```python
from build123d import *

# Parameters (mm, degrees)
BOSS_EXTRUDE2_REACH            = 37.012
BOSS_EXTRUDE2_END_MAJOR_RADIUS = 17.132631579
BOSS_EXTRUDE2_END_MINOR_RADIUS = 5.617368421
SKETCH4_W                      = 2
SKETCH4_H                      = 2
CIRPATTERN2_COUNT              = 3


with BuildPart() as part:
    # Sketch3 → Revolve1 (revolve)
    with BuildSketch(Plane.XY, mode=Mode.PRIVATE) as revolve1_sk:
        with BuildLine():
            Line((-24.25, 0), (-24.25, -1))
            ThreePointArc((-24.25, -1), (-22.452699724, -5.636404857), (-18, -7.85))
            Line((-18, -7.85), (0, -7.85))
            Line((0, -7.85), (0, -3.85))
            Line((0, -3.85), (-3.5, -3.85))
            Line((-3.5, -3.85), (-3.5, -6.35))
            Line((-3.5, -6.35), (-18, -6.35))
            ThreePointArc((-18, -6.35), (-21.400368447, -4.45256759), (-22.75, -0.8))
            Line((-22.75, -0.8), (-22.75, 0))
            Line((-22.75, 0), (-24.25, 0))
        make_face()
    revolve(revolve1_sk.sketch.rotate(Axis((0, -13.198525541, 0), (0, 1, 0)), 180), axis=Axis((0, -13.198525541, 0), (0, 1, 0)))

    # Boss-Extrude2: up to this torus (the profile starts inside it)
    boss_extrude2_end = Plane(origin=(0, -0.8, 0), z_dir=(0, -1, 0)) * Torus(BOSS_EXTRUDE2_END_MAJOR_RADIUS, BOSS_EXTRUDE2_END_MINOR_RADIUS, mode=Mode.PRIVATE)
    # Sketch4 → Boss-Extrude2 (add, up to the surface)
    with BuildSketch(Plane(origin=(0, -0.8, 0), x_dir=(1, 0, 0), z_dir=(0, 1, 0)), mode=Mode.PRIVATE) as boss_extrude2_sk1:
        with Locations((-21.75, 0)):
            Rectangle(SKETCH4_W, SKETCH4_H)
    boss_extrude2_tool1 = extrude(boss_extrude2_sk1.sketch, amount=-BOSS_EXTRUDE2_REACH, mode=Mode.PRIVATE) & boss_extrude2_end
    boss_extrude2 = boss_extrude2_tool1.solids().sort_by_distance((-21.75, -0.8, 0))[0]
    add(boss_extrude2)

    # CirPattern2: Boss-Extrude2 ×3 about axis
    cirpattern2_axis = Axis((0, 0, 0), (0, 1, 0))
    for i in range(1, CIRPATTERN2_COUNT):
        add(boss_extrude2.rotate(cirpattern2_axis, i * 360 / CIRPATTERN2_COUNT))


solid = part.part
```
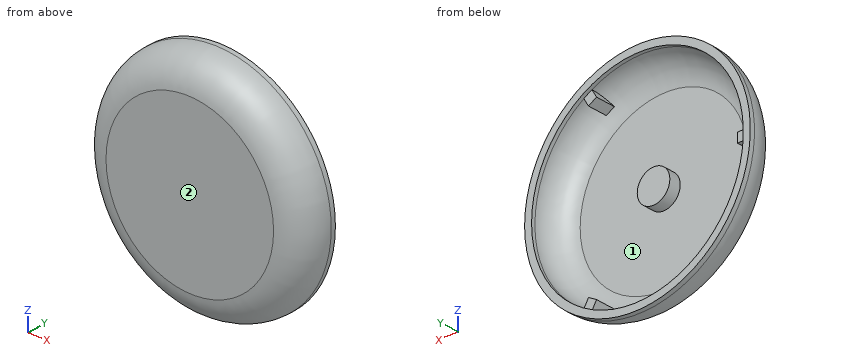
Geometry: final body of the model. Coordinates: model frame, mm. Face numbers are marked on the shaded views. A direction names the side the tool comes from. Give positions to 0.01 mm unless a question says otherwise; leave off trailing zeros. Loops run counter-clockwise (first coordinate to the right, second up) from the corner with the lowest first, then second, coordinate; pieces in that order, holes last. Notation, with made-up numbers: (29.5, -13.75) -> (57.5, -13.75) arc R11 ccw to (57.5, -4.75) -> close; hole circle Ø7 at (-16.5, 81). An arc over 180 degrees is marked (long way). Use CSV: the item, a comma, the result in double quotes.
(1) Access query for the marked faces 1 and 2. Directions: +Z, -Z, +X, -X, +Y, -Y. A direction counts if a zero-diameter tool reaches every point of the face in a straight line with its end or side. Return the directions, or none.
From the geometry:
face 1,"+Y"
face 2,"+Z, -Z, +X, -X, -Y"
(2) Cut plane B-B (y = -1.75). Output: boundary loops of the cut face in (x, z).
From the geometry:
outline,"circle Ø48.42 at (0, 0); hole (-22.65, -1) arc R22.67 ccw to (10.46, -20.11) -> (9.51, -18.47) -> (11.24, -17.47) -> (12.19, -19.11) arc R22.67 ccw to (12.19, 19.11) -> (11.24, 17.47) -> (9.51, 18.47) -> (10.46, 20.11) arc R22.67 ccw to (-22.65, 1) -> (-20.75, 1) -> (-20.75, -1) -> close"
(3) Cut plane A-A (x = 0). Output: boundary loops of the cut face in (y, z), plus the area to 3 significant figures.
From the geometry:
outline,"(-7.85, -18) arc R6.88 ccw to (-1, -24.25) -> (0, -24.25) -> (0, -22.75) -> (-0.8, -22.75) arc R5.62 cw to (-6.35, -18) -> (-6.35, -3.5) -> (-3.85, -3.5) -> (-3.85, 3.5) -> (-6.35, 3.5) -> (-6.35, 18) arc R5.62 cw to (-0.8, 22.75) -> (0, 22.75) -> (0, 24.25) -> (-1, 24.25) arc R6.88 ccw to (-7.85, 18) -> close"
area,"102 mm^2"
(4) First-contact query: P1, Ø2, axis at x = -21.5, z = 0, coming from the +Y side; P2, Ø5.5, axis at x = 1, z = 1, coming from the +Y side; P3, Ø1.6, axis at y = -2, z = 0, coming from the +X side. Flat tips, straight axial feed; report the tip coordinate or a pass-through.
From the geometry:
P1,"y = -0.8"
P2,"y = -3.85"
P3,"x = 24.25"
(5) Cut plane C-C (z = 0). Output: boundary loops of the cut face in (x, y).
From the geometry:
outline,"(-24.25, -1) arc R6.88 ccw to (-18, -7.85) -> (18, -7.85) arc R6.88 ccw to (24.25, -1) -> (24.25, 0) -> (22.75, 0) -> (22.75, -0.8) arc R5.62 cw to (18, -6.35) -> (3.5, -6.35) -> (3.5, -3.85) -> (-3.5, -3.85) -> (-3.5, -6.35) -> (-18, -6.35) arc R5.62 cw to (-20.75, -5.1) -> (-20.75, -0.8) -> (-22.75, -0.8) -> (-22.75, 0) -> (-24.25, 0) -> close"
(6) Ray query, line 1 along Z through (x, y) = (0, -0.4); line 2 along X through (y, z) = (-4, 18); line 3 along Y through (x, z) = (8, 7). Return the intervals inside material, ascending. Write a range as [from, to].
From the geometry:
line 1,"[-24.25, -22.75], [22.75, 24.25]"
line 2,"[-15.2, -12.21], [10.32, 11.55], [12.21, 15.2]"
line 3,"[-7.85, -6.35]"
